from build123d import *

# Parameters (mm, degrees)
SKETCH_1_W          = 80
SKETCH_1_H          = 80
SKETCH_1_R          = 2.65
SKETCH_1_R_2        = 1.55
EXTRUDE_1_DEPTH     = 4
SKETCH_2_R          = 1.6
CUT_EXTRUDE_1_DEPTH = 57.709787515
SKETCH_3_W          = 114.446601022
SKETCH_3_H          = 92.900037665
CUT_EXTRUDE_2_DEPTH = 1


with BuildPart() as part:
    # 草图1 → 凸台-拉伸1 (new body)
    with BuildSketch(Plane(origin=(0, 0, 0), x_dir=(1, 0, 0), z_dir=(0, 1, 0))):
        Rectangle(SKETCH_1_W, SKETCH_1_H)
        with Locations(Location((-32.5, 32.5, 0), (0, 0, 270))):
            Circle(SKETCH_1_R, mode=Mode.SUBTRACT)
        with Locations(Location((-32.5, -32.5, 0), (0, 0, 270))):
            Circle(SKETCH_1_R, mode=Mode.SUBTRACT)
        with Locations(Location((32.5, 32.5, 0), (0, 0, 270))):
            Circle(SKETCH_1_R_2, mode=Mode.SUBTRACT)
        with Locations(Location((32.5, -32.5, 0), (0, 0, 270))):
            Circle(SKETCH_1_R_2, mode=Mode.SUBTRACT)
    extrude(amount=EXTRUDE_1_DEPTH)

    # 草图2 → 切除-拉伸1 (cut, through all)
    with BuildSketch(Plane(origin=(0, 4, 0), x_dir=(1, 0, 0), z_dir=(0, 1, 0))):
        with Locations(Location((13.435028843, 13.435028843, 0), (0, 0, 270))):
            Circle(SKETCH_2_R)
        with Locations(Location((13.435028843, -13.435028843, 0), (0, 0, 270))):
            Circle(SKETCH_2_R)
        with Locations(Location((-13.435028843, -13.435028843, 0), (0, 0, 270))):
            Circle(SKETCH_2_R)
        with Locations(Location((-13.435028843, 13.435028843, 0), (0, 0, 270))):
            Circle(SKETCH_2_R)
    extrude(amount=-CUT_EXTRUDE_1_DEPTH, mode=Mode.SUBTRACT)

    # 草图3 → 切除-拉伸2 (cut)
    with BuildSketch(Plane.XZ):
        with Locations((9.368071025, -1.951681463)):
            Rectangle(SKETCH_3_W, SKETCH_3_H)
    extrude(amount=-CUT_EXTRUDE_2_DEPTH, mode=Mode.SUBTRACT)


solid = part.part
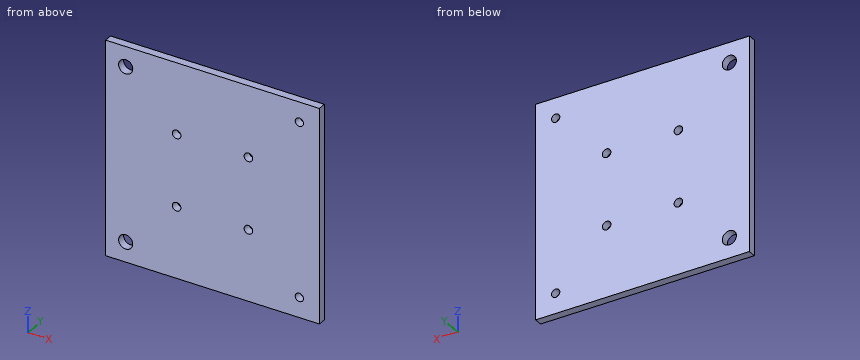
Design review of the part built by this model. Coordinates are the model's own, in mm. Give positions to 0.01 mm unless a question says otherwise; leave off trailing zeros. Order: outer loops, then holes, each group sorted by start corner. A loop starts at its lowest first (then second) coordinate and runs counter-clockwise, first axis right, second up.
1. For pin 1 Ø8.5 at (x, z) = (-32.5, -32.5) entering from -Y, flat-tipped, find the tip position at first contact; note if it passes through.
Solution:
pin 1: stops at y = 1
2. Add section B-B, the plane z = 32.5. State the section outline as (x, y) points.
Solution:
outline: (-40, 1) - (-35.15, 1) - (-35.15, 4) - (-40, 4) - close; (-29.85, 1) - (30.95, 1) - (30.95, 4) - (-29.85, 4) - close; (34.05, 1) - (40, 1) - (40, 4) - (34.05, 4) - close
3. Add section A-A, the plane x = 32.5. State the section outline as (y, z) points.
Solution:
outline: (1, -40) - (4, -40) - (4, -34.05) - (1, -34.05) - close; (1, -30.95) - (4, -30.95) - (4, 30.95) - (1, 30.95) - close; (1, 34.05) - (4, 34.05) - (4, 40) - (1, 40) - close
4. To check wall thickness, follow L1, parallel to X at y = 3.25, z = -32.5; L2, parallel to Z at x = -32.5, y = 1.9; L3, parallel to X at y = 1.7, z = 13. State the ranges of each line that lie inside material, in increasing order.
Solution:
L1: x = -40 to -35.15, -29.85 to 30.95, 34.05 to 40
L2: z = -40 to -35.15, -29.85 to 29.85, 35.15 to 40
L3: x = -40 to -14.97, -11.9 to 11.9, 14.97 to 40
